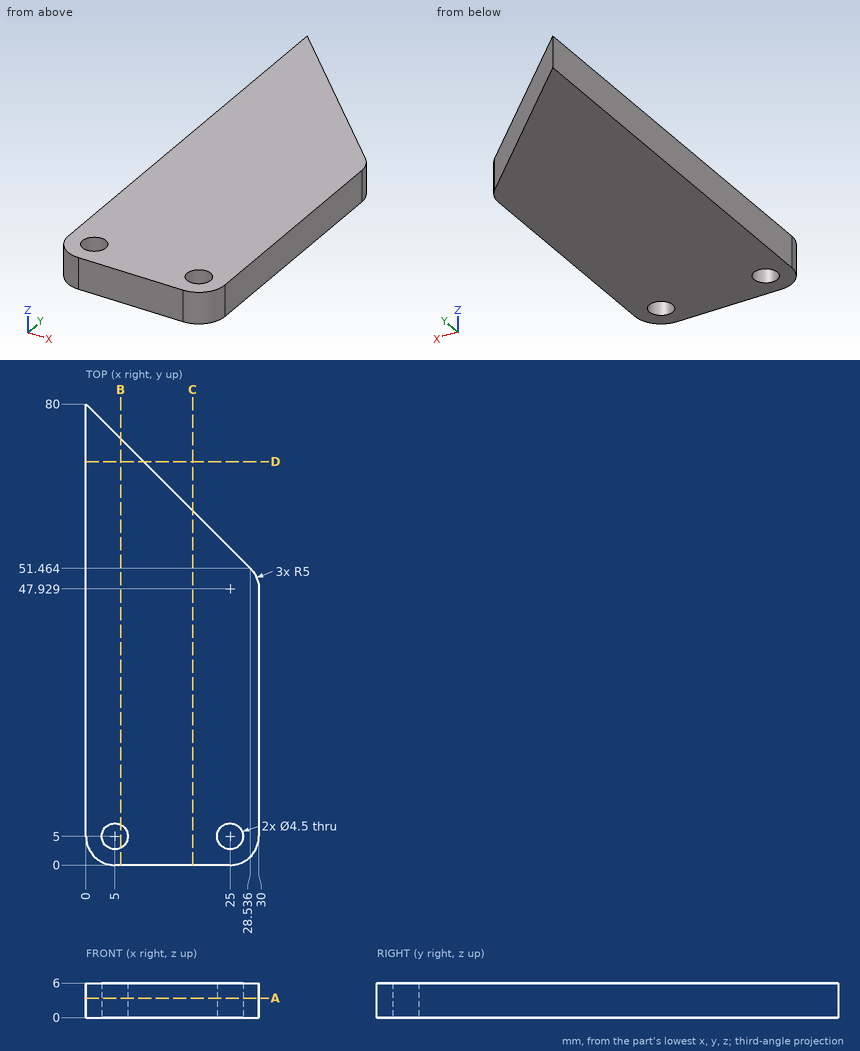
Here's the drawing with two shaded views (mm, measured from the low corner). I have some questions. Give positions to 0.01 mm unless a question says otherwise; leave off trailing zeros. Order: outer loops, then holes, each group sorted by start corner. A loop starts at its lowest first (then second) coordinate and runs counter-clockwise, first axis right, second up.
Q1. Suppose I cut it at D-D, the plane y = 70. Write out the boundary of the cut face in (x, z), and give its area (3 significant figures).
Q2. Suppose I cut it at C-C, the plane x = 18.5. Write out the boundary of the cut face in (y, z).
Q3. I'm going to push a flat-ended pin straight in: P1, Ø4, axis at x = 5, y = 5, coming from the +Z side. Where does the tip first touch, or does it pass through?
Q4. If I drill on line 1 along Y through (x, z) = (25, 3.9); line 2 along Y through (x, z) = (5, 1.9); line 3 along Y through (x, z) = (18, 3.3), over which ranges is the centre line in solid material (lowest first)?
Q5. Suppose I cut it at A-A, the plane z = 3.4. Count the separate pieces of the cut face and the enclosed holes in it, and give its area (3 significant figures).
Q6. Suppose I cut it at B-B, the plane x = 6. Write out the boundary of the cut face in (y, z) (1 decimal).
Solution:
1. outline: (0, 0) - (10, 0) - (10, 6) - (0, 6) - close
1. area: 60.0 mm2
2. outline: (0, 0) - (61.5, 0) - (61.5, 6) - (0, 6) - close
3. P1: passes through
4. line 1: y = 0 to 2.75, 7.25 to 55
4. line 2: y = 0 to 2.75, 7.25 to 75
4. line 3: y = 0 to 62
5. separate pieces: 1
5. enclosed holes: 2
5. area: 1,910 mm2
6. outline: (0, 0) - (3, 0) - (3, 6) - (0, 6) - close; (7, 0) - (74, 0) - (74, 6) - (7, 6) - close
